The listing builds one solid part. Answer for the finished solid, in the listing's coordinates (mm). Round coordinates to 2 decimals unless told otherwise and drop trailing zeros. Return JSON: item names as keys, results as strings. Group by question number.
from build123d import *

# Parameters (mm, degrees)
F1_R = 4


with BuildPart() as f2:
    # F2: sweep along a path in F0
    with BuildLine(Plane.XZ) as f2_path:
        Line((0, 0), (-21, 0))
        ThreePointArc((-21, 0), (-24.535534, 1.464466), (-26, 5))
        Line((-26, 5), (-26, 91))
        ThreePointArc((-26, 91), (-24.535534, 94.535534), (-21, 96))
        Line((-21, 96), (0, 96))
    # F1 (on Right) → F2 (sweep)
    with BuildSketch(Plane.YZ):
        Circle(F1_R)
    sweep(path=f2_path.line)


solid = f2.part
(1) Determine the mould class of faces 1 (the cylindrical face through (-10.647, -0.867, 3.905)), 2 (the flat face through (0, 0, 96)) for opening direction Z: +Z half, -Z half, draft (parallel to the pull), parting line (faces both ways), or undercut.
(2) Flat-ended cylindrical pins translate along their axes: pin 1 (2 mm diameter, centred on y = 1.5, z = 66, fed in from -X); pin 2 (1 mm diameter, centred on x = -14.5, y = 1, fed in from -Z); pin 3 (4 mm diameter, centred on x = -7, y = 3, fed in from +Z). Find the tip coordinate at first contact, or state that the pin passes through.
(3) Consider line 1 (Z direction, x = -2.5, y = 0.25); line 2 (Z direction, x = -12.5, y = -0.75); line 3 (X direction, y = 0.25, z = 64). Determine where each line is inside the solid, lowest interval first.
Check sheet entries:
{
 "1": {"face 1": "undercut", "face 2": "draft"},
 "2": {"pin 1": "stops at x = -29.97", "pin 2": "stops at z = -3.97", "pin 3": "stops at z = 99.87"},
 "3": {"line 1": "z = -3.99 to 3.99, 92.01 to 99.99", "line 2": "z = -3.93 to 3.93, 92.07 to 99.93", "line 3": "x = -29.99 to -22.01"}
}
